Could you check a few things on this drawing? It's one solid part, dimensions in mm from its lowest x, y, z. A direction names the side the tool comes from. Give positions to 0.01 mm unless a question says otherwise; leave off trailing zeros. Order: outer loops, then holes, each group sorted by start corner. A loop starts at its lowest first (then second) coordinate and runs counter-clockwise, first axis right, second up. Notation, with made-up numbers: (-37, 3.25) - (16, 3.25) arc R28 cw to (16, 23.25) - close; hole circle Ø7 at (9, 67). An arc over 180 degrees is marked (long way). One line per question, with ' | ' between items. Start each with the question number.
1. I need wall thicknesses on probe 1 along X at (y, z) = (7.75, 21); probe 2 along Z at (x, y) = (9.25, 5.5); probe 3 along Y at (x, z) = (54, 1). Which ranges of each line are inside material? Lowest first, please. Write a range as from..to.
2. For P1, Ø5.5, axis at x = 5, y = 7, coming from the +Z side; P2, Ø2, axis at y = 10.5, z = 36, coming from the -X side; P3, Ø9, axis at x = 30, z = 21, coming from the +Y side, each with a flat end and sliding along its axis, tell me the tip position at first contact or that it passes through.
3. Imagine slicing it at B-B (z = 5). Please give me the cut outline in (x, y), and give its area (3 significant figures).
4. Imagine slicing it at C-C (x = 36). Please give me the cut outline in (y, z), and give its area (3 significant figures).
5. Imagine slicing it at A-A (y = 11). Please give me the cut outline in (x, z).
6. Imagine slicing it at D-D (y = 6). Give the number of separate pieces and of enclosed holes in the cut face, and give its area (3 significant figures).
7. Which directions (+Z, -Z, +X, -X, +Y, -Y) give clear straight access to the entire face, cutting with the end or side of a thin tool? Please do the marked faces 4, 5 and 6.
8. If we mould it in two halves opening along X, with no side actions, what happens to the marked faces 1, 2 and 3? For each: released by +X, released by -X, zero draft, split by the parting line, or undercut.
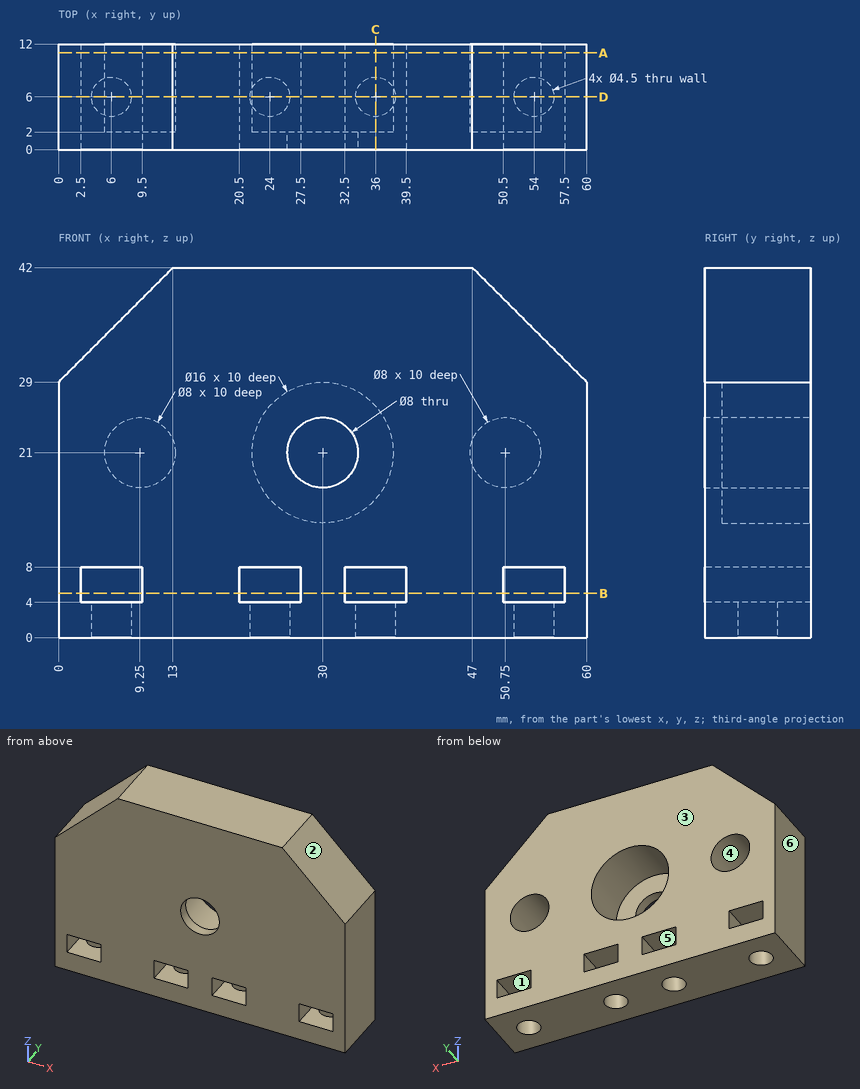
Results found:
1) probe 1: x = 0..5.25, 13.25..22, 38..46.75, 54.75..60 | probe 2: z = 0..4, 8..17, 25..38.25 | probe 3: y = 0..3.75, 8.25..12
2) P1: stops at z = 36.75 | P2: stops at x = 6 | P3: stops at y = 2
3) outline: (0, 0) - (2.5, 0) - (2.5, 12) - (0, 12) - close; (9.5, 0) - (20.5, 0) - (20.5, 12) - (9.5, 12) - close; (27.5, 0) - (32.5, 0) - (32.5, 12) - (27.5, 12) - close; (39.5, 0) - (50.5, 0) - (50.5, 12) - (39.5, 12) - close; (57.5, 0) - (60, 0) - (60, 12) - (57.5, 12) - close | area: 384 mm2
4) outline: (0, 0) - (3.75, 0) - (3.75, 4) - (0, 4) - close; (0, 8) - (12, 8) - (12, 15.71) - (2, 15.71) - (2, 26.29) - (12, 26.29) - (12, 42) - (0, 42) - close; (8.25, 0) - (12, 0) - (12, 4) - (8.25, 4) - close | area: 332 mm2
5) outline: (0, 0) - (60, 0) - (60, 29) - (47, 42) - (13, 42) - (0, 29) - close; hole (2.5, 4) - (9.5, 4) - (9.5, 8) - (2.5, 8) - close; hole circle Ø8 at (9.25, 21); hole (20.5, 4) - (27.5, 4) - (27.5, 8) - (20.5, 8) - close; hole circle Ø16 at (30, 21); hole (32.5, 4) - (39.5, 4) - (39.5, 8) - (32.5, 8) - close; hole circle Ø8 at (50.75, 21); hole (50.5, 4) - (57.5, 4) - (57.5, 8) - (50.5, 8) - close
6) separate pieces: 1 | enclosed holes: 3 | area: 1,870 mm2
7) face 4: +Y | face 5: +Y, -Y | face 6: +Z, -Z, -X, +Y, -Y
8) face 1: undercut | face 2: released by +X | face 3: zero draft
